```python
from build123d import *

# Parameters (mm, degrees)
F0_W     = 20
F0_H     = 20
F1_DEPTH = 10
F2_R     = 5
F3_DEPTH = 30


with BuildPart() as f1:
    # F0 (on Top) → F1 (new body)
    with BuildSketch(Plane.XY):
        Rectangle(F0_W, F0_H)
    extrude(amount=F1_DEPTH)

    # F2 (on face) → F3 (join)
    with BuildSketch(Plane.YZ.offset(10)):
        with Locations((0, 13.975238)):
            Circle(F2_R)
    extrude(amount=-F3_DEPTH)


solid = f1.part
```
The listing builds one solid part. Answer for the finished solid, in the listing's coordinates (mm). A direction names the side the tool comes from. Give positions to 0.01 mm unless a question says otherwise; leave off trailing zeros. Write each loop counter-clockwise with the first axis right and the second up, starting at its lowest first coordinate (ties: lowest second). Pieces come first, ordered by that corner, then holes. Notation, with made-up numbers: (38, 15.25) - (84, 15.25) arc R25 cw to (84, 49.25) - close; hole circle Ø8 at (12.25, 76). An arc over 180 degrees is marked (long way). Use one line per item in the form item = value. Start each with the question number.
1) Find section D-D on z = 3. Determine the outline of the cut face in (x, y), plus the area to 3 significant figures.
2) Find section B-B on x = -9.25. Determine the outline of the cut face in (y, z).
3) Find section C-C on y = 0. Determine the outline of the cut face in (x, z).
4) Consider line 1 along Z through (x, y) = (7.5, 7.5); line 2 along X through (y, z) = (6.75, 8.5); line 3 along Y through (x, z) = (-17.75, 14.25). Determine where each line is inside the solid, lowest interval first. Write a range as from..to.
5) A tool of negligible diameter and unlimited length cuts with its end or side. For faces 1 (the face through (0, 7, 10)), 2 (the face through (10, 0, 8)), from which of +Z, -Z, +X, -X, +Y, -Y can it reach the whole face along a straight path? Write none if from no direction.
6) Flat-ended cylindrical pins translate along their axes: pin 1 Ø8 at (y, z) = (-0.5, 4.5) entering from -X; pin 2 Ø1 at (x, y) = (-12.5, -1.5) entering from -Z; pin 3 Ø5.5 at (x, y) = (3, -6.5) entering from +Z. Find the tip coordinate at first contact, or state that the pin passes through.
7) Find section A-A on y = -4.25. Determine the outline of the cut face in (x, z), plus the area to 3 significant figures.
Geometry results:
q1.outline = (-10, -10) - (10, -10) - (10, 10) - (-10, 10) - close
q1.area = 400 mm2
q2.outline = (-10, 0) - (10, 0) - (10, 10) - (3.03, 10) arc R5 ccw (long way) to (-3.03, 10) - (-10, 10) - close
q3.outline = (-20, 8.98) - (-10, 8.98) - (-10, 0) - (10, 0) - (10, 18.98) - (-20, 18.98) - close
q4.line_1 = 0..10
q4.line_2 = -10..10
q4.line_3 = -4.99..4.99
q5.face_1 = +X, -X, +Y
q5.face_2 = +Z, -Z, +X, +Y, -Y
q6.pin_1 = -10
q6.pin_2 = 9.08
q6.pin_3 = 17.28
q7.outline = (-20, 11.34) - (10, 11.34) - (10, 16.61) - (-20, 16.61) - close; (-10, 0) - (10, 0) - (10, 10) - (-10, 10) - close
q7.area = 358 mm2
